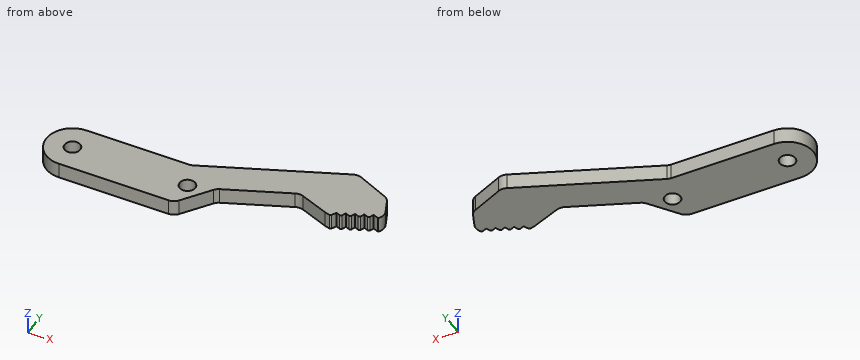
```python
from build123d import *

# Parameters (mm, degrees)
SKETCH2_R           = 1.5
BOSS_EXTRUDE1_DEPTH = 3
FILLET1_START       = -1
FILLET1_DEPTH       = 5
FILLET1_2_DEPTH     = 3
FILLET2_R           = 0.3


with BuildPart() as part:
    # Sketch2 → Boss-Extrude1 (new body)
    with BuildSketch(Plane.XY):
        with BuildLine():
            Line((20.05, 5), (0, 5))
            ThreePointArc((0, 5), (-5, 0), (0, -5))
            Line((0, -5), (22, -5))
            Line((22, -5), (26.795441544, 1.415535375))
            Line((26.795441544, 1.415535375), (39.960977063, 6.841977535))
            Line((39.960977063, 6.841977535), (45.957673933, 4.467717283))
            Line((45.957673933, 4.467717283), (47.183545432, 4.117717283))
            Line((47.183545432, 4.117717283), (47.806766001, 5.229858036))
            Line((47.806766001, 5.229858036), (48.839161842, 4.800113125))
            Line((48.839161842, 4.800113125), (49.268906753, 5.832508966))
            Line((49.268906753, 5.832508966), (50.301302595, 5.402764054))
            Line((50.301302595, 5.402764054), (50.731047506, 6.435159896))
            Line((50.731047506, 6.435159896), (51.763443347, 6.005414984))
            Line((51.763443347, 6.005414984), (52.193188259, 7.037810826))
            Line((52.193188259, 7.037810826), (53.2255841, 6.608065914))
            Line((53.2255841, 6.608065914), (53.655329011, 7.640461756))
            Line((53.655329011, 7.640461756), (54.687724853, 7.210716844))
            Line((54.687724853, 7.210716844), (55.741112884, 7.640461756))
            Line((55.741112884, 7.640461756), (55.434270778, 8.373688641))
            Line((55.434270778, 8.373688641), (53.719454084, 12.534145792))
            Line((53.719454084, 12.534145792), (46.399561958, 15.860505726))
            Line((46.399561958, 15.860505726), (20.05, 5))
        make_face()
        Circle(SKETCH2_R, mode=Mode.SUBTRACT)
        with Locations((22, 0)):
            Circle(SKETCH2_R, mode=Mode.SUBTRACT)
    extrude(amount=BOSS_EXTRUDE1_DEPTH)

    # Fillet1: read off the stored shape, not the designer's step
    # Fillet1 outline → Fillet1 (cut)
    with BuildSketch(Plane.XY.offset(FILLET1_START)):
        with BuildLine():
            Line((55.434270778, 8.373688641), (55.048718881, 9.309107658))
            ThreePointArc((55.048718881, 9.309107658), (55.170672337, 8.207880564), (54.687724853, 7.210716844))
            Line((54.687724853, 7.210716844), (55.741112884, 7.640461756))
            Line((55.741112884, 7.640461756), (55.434270778, 8.373688641))
        make_face()
        with BuildLine():
            Line((53.719454084, 12.534145792), (52.999247687, 12.861427351))
            ThreePointArc((52.999247687, 12.861427351), (53.610964364, 12.429448634), (54.020911938, 11.802754217))
            Line((54.020911938, 11.802754217), (53.719454084, 12.534145792))
        make_face()
        with BuildLine():
            Line((46.399561958, 15.860505726), (45.598653524, 15.530395091))
            ThreePointArc((45.598653524, 15.530395091), (46.396368341, 15.68098662), (47.188222093, 15.50211691))
            Line((47.188222093, 15.50211691), (46.399561958, 15.860505726))
        make_face()
        with BuildLine():
            Line((22, -5), (22.59991613, -4.197407971))
            ThreePointArc((22.59991613, -4.197407971), (21.893850393, -4.788129741), (20.997975386, -5))
            Line((20.997975386, -5), (22, -5))
        make_face()
    extrude(amount=FILLET1_DEPTH, mode=Mode.SUBTRACT)

    # Fillet1 2 outline → Fillet1 2 (add)
    with BuildSketch(Plane.XY):
        with BuildLine():
            ThreePointArc((20.416130089, 5.150907933), (20.042458039, 5.038089689), (19.653989336, 5))
            Line((19.653989336, 5), (20.05, 5))
            Line((20.05, 5), (20.416130089, 5.150907933))
        make_face()
        with BuildLine():
            ThreePointArc((26.465363358, 0.973943448), (26.841174676, 1.356600864), (27.305163351, 1.625627544))
            Line((27.305163351, 1.625627544), (26.795441544, 1.415535375))
            Line((26.795441544, 1.415535375), (26.465363358, 0.973943448))
        make_face()
        with BuildLine():
            ThreePointArc((39.213895373, 6.534052683), (39.962073605, 6.684911877), (40.712285231, 6.544513587))
            Line((40.712285231, 6.544513587), (39.960977063, 6.841977535))
            Line((39.960977063, 6.841977535), (39.213895373, 6.534052683))
        make_face()
    extrude(amount=FILLET1_2_DEPTH)

    # Fillet2
    fillet2_edges = [part.edges().sort_by_distance(p)[0] for p in [
        (53.2255841, 6.608065914, 1.5),
        (51.763443347, 6.005414984, 1.5),
        (50.301302595, 5.402764054, 1.5),
        (48.839161842, 4.800113125, 1.5),
        (47.183545432, 4.117717283, 1.5),
    ]]
    fillet(fillet2_edges, radius=FILLET2_R)


solid = part.part
```
For this review, take the finished solid that the model builds, in its own axes (mm). Round coordinates to 2 decimals unless told otherwise and drop trailing zeros. Write each loop counter-clockwise with the first axis right and the second up, starting at its lowest first coordinate (ties: lowest second). Pieces come first, ordered by that corner, then holes. Notation, with made-up numbers: (83.5, 87.25) - (139.5, 87.25) arc R16 cw to (139.5, 104.25) - close; hole circle Ø2 at (-33.5, -11). An arc over 180 degrees is marked (long way). Answer as CSV lines item,"result". Start each with the question number.
(1) Add section C-C, the plane y = 0. State the section outline as (x, z) points.
(2) Add section B-B, the plane x = 22. State the section outline as (y, z) points, plus the area to 3 significant figures.
(3) Add section A-A, the plane z = 0.7. State how many separate pieces and enclosed holes the cut face has, plus the area to 3 significant figures.
(4) For pin 1 (10 mm diameter, centred on x = 42, y = 5, fed in from +Z), flat-tipped, find the tip position at first contact; note if it passes through.
(5) Add section D-D, the plane x = 5.5. State the section outline as (y, z) points.
(6) For line 1 (Y direction, x = 0, z = 2.15); line 2 (X direction, y = 1, z = 0.3); line 3 (Y direction, x = 4, z = 1.95), list the stretches that pass through material, from the lowest coordinate up.
From the geometry:
1,outline,"(-5, 0) - (-1.5, 0) - (-1.5, 3) - (-5, 3) - close; (1.5, 0) - (20.5, 0) - (20.5, 3) - (1.5, 3) - close; (23.5, 0) - (25.74, 0) - (25.74, 3) - (23.5, 3) - close"
2,outline,"(-4.73, 0) - (-1.5, 0) - (-1.5, 3) - (-4.73, 3) - close; (1.5, 0) - (5.8, 0) - (5.8, 3) - (1.5, 3) - close"
2,area,"22.6 mm²"
3,separate pieces,"1"
3,enclosed holes,"2"
3,area,"495 mm²"
4,pin 1,"stops at z = 3"
5,outline,"(-5, 0) - (5, 0) - (5, 3) - (-5, 3) - close"
6,line 1,"y = -5 to -1.5, 1.5 to 5"
6,line 2,"x = -4.9 to -1.12, 1.12 to 20.88, 23.12 to 26.49"
6,line 3,"y = -5 to 5"
